Autodesk Fusion 360 part; units mm, degrees
sketch "Skizze1" plane through (0, 0, 0) normal (0, 0, 1) x (1, 0, 0)
  line L0 (0, 0) -> (100, 0)
  line L1 (100, 0) -> (100, 100)
  line L2 (100, 100) -> (0, 100)
  line L3 (0, 100) -> (0, 0)
  line L4 (100, 100) -> (20, 100)
  line L5 (20, 100) -> (20, 20)
  line L6 (20, 20) -> (100, 20)
  line L7 (100, 20) -> (100, 100)
  circle A0 centre (96, 24) radius 2
  circle A1 centre (24, 96) radius 2
  circle A2 centre (96, 96) radius 2
  circle A3 centre (24, 24) radius 2
  circle A4 centre (60, 60) radius 34.5
  dimension "d1" = 100
  dimension "d2" = 100
  dimension "d3" = 80
  dimension "d4" = 80
  dimension "d5" = 72
  dimension "d6" = 72
  dimension "d9" = 4
  dimension "d10" = 4
  dimension "d11" = 4
  dimension "d12" = 4
  dimension "d13" = 69
extrude "Extrusion1" add sketch "Skizze1" along normal blind 3
sketch "Skizze2" plane through (0, 0, 3) normal (0, 0, 1) x (-1, 0, 0)
  circle A0 centre (-24, -24) radius 2
  circle A1 centre (-60, -60) radius 34.5
  circle A2 centre (-96, -24) radius 2
  circle A3 centre (-96, -96) radius 2
  circle A4 centre (-24, -96) radius 2
  line L0 (-100, 0) -> (-100, -100)
  line L1 (-100, -100) -> (0, -100)
  line L2 (0, -100) -> (0, 0)
  line L3 (0, 0) -> (-100, 0)
  circle A5 centre (-95, -10) radius 1.6
  circle A6 centre (-20, -10) radius 1.6
  circle A7 centre (-10, -20) radius 1.6
  circle A8 centre (-10, -95) radius 1.6
  dimension "d17" = 3.2
  dimension "d18" = 3.2
  dimension "d19" = 3.2
  dimension "d20" = 3.2
extrude "Extrusion2" cut sketch "Skizze2" against normal blind 10 contours A5 | A6 | A7 | A8
sketch "Skizze3" plane through (0, 0, 3) normal (0, 0, 1) x (-1, 0, 0)
  circle A0 centre (-10, -20) radius 1.6
  circle A1 centre (-95, -10) radius 1.6
  circle A2 centre (-20, -10) radius 1.6
  circle A3 centre (-10, -95) radius 1.6
  circle A4 centre (-96, -96) radius 2
  circle A5 centre (-24, -24) radius 2
  circle A6 centre (-24, -96) radius 2
  circle A7 centre (-60, -60) radius 34.5
  circle A8 centre (-96, -24) radius 2
  line L0 (-100, 0) -> (-100, -100)
  line L1 (-100, -100) -> (0, -100)
  line L2 (0, -100) -> (0, 0)
  line L3 (0, 0) -> (-100, 0)
  circle A9 centre (-60, -60) radius 36.5
  dimension "d23" = 73
extrude "Extrusion3" add sketch "Skizze3" along normal blind 30 contours A9
Geometry check sheet. Reference: the model listing, model coordinates, mm. A direction names the side the tool comes from. Coordinates: 2 decimals unless noted, no trailing zeros. Loops run counter-clockwise (first coordinate to the right, second up) from the corner with the lowest first, then second, coordinate; pieces in that order, holes last.
Item 1: Release check for a two-part mould opening along X. For faces 1 (the face through (27, 40, 0)), 2 (the face through (100, 49, 1)), 3 (the face through (96.6, 9.93, 1.52)) record: released by +X, released by -X, zero draft, split by the parting line, or undercut.
Item 2: Sectioned sample at A-A, the plane y = 60. Record the boundary of the cut face in (x, z), then the cut area to 3 significant figures.
Item 3: Sectioned sample at C-C, the plane z = 27.5. Record the boundary of the cut face in (x, y).
Item 4: Go/stop test with flat-tipped pins: pin 1 Ø6.5 at (x, y) = (96, 96) entering from +Z; pin 2 Ø4.5 at (x, y) = (96, 24) entering from -Z; pin 3 Ø6 at (x, z) = (58, 27.5) entering from +Y; pin 4 Ø2 at (x, z) = (82, 29) entering from +Y. Record where each tip stops, or that it passes through.
Item 5: Sectioned sample at D-D, the plane x = 20. Record the boundary of the cut face in (y, z), then the cut area to 3 significant figures.
Item 6: Access from +Z, -Z, +X, -X, +Y, -Y to the whole of each face (thin tool, end or side, straight path). Record for faces 4 (the face through (27, 40, 3)), 5 (the face through (51, 100, 1)).
Item 7: Thickness scan on line 1 (X direction, y = 10, z = 1); line 2 (Y direction, x = 20, z = 0.95); line 3 (X direction, y = 60, z = 1). Record the ranges inside material, lowest first.
Check result:
1. face 1: zero draft
1. face 2: released by +X
1. face 3: undercut
2. outline: (0, 0) - (25.5, 0) - (25.5, 33) - (23.5, 33) - (23.5, 3) - (0, 3) - close; (94.5, 0) - (100, 0) - (100, 3) - (96.5, 3) - (96.5, 33) - (94.5, 33) - close
2. area: 213 mm2
3. outline: circle Ø73 at (60, 60); hole circle Ø69 at (60, 60)
4. pin 1: stops at z = 3
4. pin 2: stops at z = 0
4. pin 3: stops at y = 96.5
4. pin 4: stops at y = 89.85
5. outline: (0, 0) - (8.4, 0) - (8.4, 3) - (0, 3) - close; (11.6, 0) - (100, 0) - (100, 3) - (11.6, 3) - close
5. area: 290 mm2
6. face 4: +Z
6. face 5: +Z, -Z, +X, -X, +Y
7. line 1: x = 0 to 18.4, 21.6 to 93.4, 96.6 to 100
7. line 2: y = 0 to 8.4, 11.6 to 100
7. line 3: x = 0 to 25.5, 94.5 to 100
